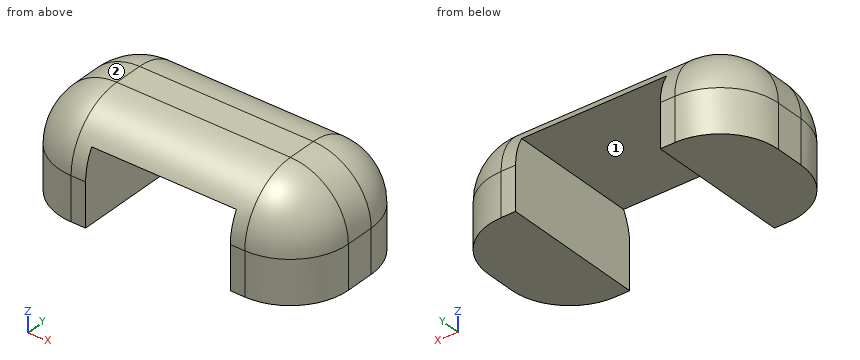
```python
from build123d import *

# Parameters (mm, degrees)
F0_W         = 5
F0_H         = 10
F1_DEPTH     = 5
F2_W         = 20
F2_H         = 10
F3_DEPTH     = 2
F4_T1_DEPTH  = 2
F4_T3_DEPTH  = 12
F4_T5_DEPTH  = 13
F4_S9_W      = 4
F4_S9_H      = 4
F4_T10_DEPTH = 4
F4_S15_W     = 4
F4_S15_H     = 4
F4_T16_DEPTH = 4
F4_S21_W     = 4
F4_S21_H     = 4
F4_T22_DEPTH = 4
F4_S27_W     = 4
F4_S27_H     = 4
F4_T28_DEPTH = 4


# Not quite as in the source:
# - a fillet or chamfer that OpenCascade refuses, or shapes differently, is made with other operations: its cross-section is extruded or revolved along the edge and cut away or added


with BuildPart() as f1:
    # F0 (on Top) → F1 (new body)
    with BuildSketch(Plane.XY):
        with Locations((-7.5, 0)):
            Rectangle(F0_W, F0_H)
    extrude(amount=F1_DEPTH)



with BuildPart() as f1b:
    # F0 (on Top) → F1, piece 2 (new body)
    with BuildSketch(Plane.XY):
        with Locations((7.5, 0)):
            Rectangle(F0_W, F0_H)
    extrude(amount=F1_DEPTH)


with BuildPart() as f1_1:
    add(f1.part)

    add(f1b.part)  # F3 merges F1b
    # F2 (on face) → F3 (join)
    with BuildSketch(Plane.XY.offset(5)):
        Rectangle(F2_W, F2_H)
    extrude(amount=F3_DEPTH)

    # F4: fillet of radius 4 on 8 edges, made by hand

    # F4_s2 → F4_t1 (cut)
    with BuildSketch(Plane.XZ.offset(-1)):
        with BuildLine():
            ThreePointArc((-10, 3), (-8.8284271247, 5.8284271247), (-6, 7))
            Line((-6, 7), (-10, 7))
            Line((-10, 7), (-10, 3))
        make_face()
        with BuildLine():
            ThreePointArc((6, 7), (8.8284271247, 5.8284271247), (10, 3))
            Line((10, 3), (10, 7))
            Line((10, 7), (6, 7))
        make_face()
    extrude(amount=F4_T1_DEPTH, mode=Mode.SUBTRACT)

    # F4_s4 → F4_t3 (cut)
    with BuildSketch(Plane.YZ.offset(-6)):
        with BuildLine():
            ThreePointArc((-5, 3), (-3.8284271247, 5.8284271247), (-1, 7))
            Line((-1, 7), (-5, 7))
            Line((-5, 7), (-5, 3))
        make_face()
        with BuildLine():
            ThreePointArc((5, 3), (3.8284271247, 5.8284271247), (1, 7))
            Line((1, 7), (5, 7))
            Line((5, 7), (5, 3))
        make_face()
    extrude(amount=F4_T3_DEPTH, mode=Mode.SUBTRACT)

    # F4_s6 → F4_t5 (cut)
    with BuildSketch(Plane.XY.offset(-10)):
        with BuildLine():
            ThreePointArc((6, -5), (8.8284271247, -3.8284271247), (10, -1))
            Line((10, -1), (10, -5))
            Line((10, -5), (6, -5))
        make_face()
        with BuildLine():
            ThreePointArc((6, 5), (8.8284271247, 3.8284271247), (10, 1))
            Line((10, 1), (10, 5))
            Line((10, 5), (6, 5))
        make_face()
        with BuildLine():
            ThreePointArc((-6, 5), (-8.8284271247, 3.8284271247), (-10, 1))
            Line((-10, 1), (-10, 5))
            Line((-10, 5), (-6, 5))
        make_face()
        with BuildLine():
            ThreePointArc((-6, -5), (-8.8284271247, -3.8284271247), (-10, -1))
            Line((-10, -1), (-10, -5))
            Line((-10, -5), (-6, -5))
        make_face()
    extrude(amount=F4_T5_DEPTH, mode=Mode.SUBTRACT)


with BuildPart() as f4_tool8:
    # F4_s9 → F4_t10 (new body)
    with BuildSketch(Plane.XY.offset(3)):
        with Locations((-8, 3)):
            Rectangle(F4_S9_W, F4_S9_H)
    extrude(amount=F4_T10_DEPTH)

    # F4_s11 → F4_t12 (revolve, cut)
    with BuildSketch(Plane(origin=(-6, 1, 3), x_dir=(0.7071067812, -0.7071067812, 0), z_dir=(-0.7071067812, -0.7071067812, 0))):
        with BuildLine():
            ThreePointArc((0, -4), (4, 0), (0, 4))
            Line((0, 4), (0, -4))
        make_face()
    revolve(axis=Axis((-6, 1, 3), (0, 0, 1)), mode=Mode.SUBTRACT)


with BuildPart() as f1_2:
    add(f1_1.part)

    # F4_t7: cut F4_tool8
    add(f4_tool8.part, mode=Mode.SUBTRACT)


with BuildPart() as f4_tool14:
    # F4_s15 → F4_t16 (new body)
    with BuildSketch(Plane.XY.offset(3)):
        with Locations((-8, -3)):
            Rectangle(F4_S15_W, F4_S15_H)
    extrude(amount=F4_T16_DEPTH)

    # F4_s17 → F4_t18 (revolve, cut)
    with BuildSketch(Plane(origin=(-6, -1, 3), x_dir=(0.7071067812, 0.7071067812, 0), z_dir=(0.7071067812, -0.7071067812, 0))):
        with BuildLine():
            ThreePointArc((0, -4), (4, 0), (0, 4))
            Line((0, 4), (0, -4))
        make_face()
    revolve(axis=Axis((-6, -1, 3), (0, 0, 1)), mode=Mode.SUBTRACT)


with BuildPart() as f1_3:
    add(f1_2.part)

    # F4_t13: cut F4_tool14
    add(f4_tool14.part, mode=Mode.SUBTRACT)


with BuildPart() as f4_tool20:
    # F4_s21 → F4_t22 (new body)
    with BuildSketch(Plane.XY.offset(3)):
        with Locations((8, -3)):
            Rectangle(F4_S21_W, F4_S21_H)
    extrude(amount=F4_T22_DEPTH)

    # F4_s23 → F4_t24 (revolve, cut)
    with BuildSketch(Plane(origin=(6, -1, 3), x_dir=(-0.7071067812, 0.7071067812, 0), z_dir=(0.7071067812, 0.7071067812, 0))):
        with BuildLine():
            ThreePointArc((0, -4), (4, 0), (0, 4))
            Line((0, 4), (0, -4))
        make_face()
    revolve(axis=Axis((6, -1, 3), (0, 0, 1)), mode=Mode.SUBTRACT)


with BuildPart() as f1_4:
    add(f1_3.part)

    # F4_t19: cut F4_tool20
    add(f4_tool20.part, mode=Mode.SUBTRACT)


with BuildPart() as f4_tool26:
    # F4_s27 → F4_t28 (new body)
    with BuildSketch(Plane.XY.offset(3)):
        with Locations((8, 3)):
            Rectangle(F4_S27_W, F4_S27_H)
    extrude(amount=F4_T28_DEPTH)

    # F4_s29 → F4_t30 (revolve, cut)
    with BuildSketch(Plane(origin=(6, 1, 3), x_dir=(-0.7071067812, -0.7071067812, 0), z_dir=(-0.7071067812, 0.7071067812, 0))):
        with BuildLine():
            ThreePointArc((0, -4), (4, 0), (0, 4))
            Line((0, 4), (0, -4))
        make_face()
    revolve(axis=Axis((6, 1, 3), (0, 0, 1)), mode=Mode.SUBTRACT)


with BuildPart() as f1_5:
    add(f1_4.part)

    # F4_t25: cut F4_tool26
    add(f4_tool26.part, mode=Mode.SUBTRACT)


solid = f1_5.part
```
The model under review builds one solid part; all positions refer to its coordinate system, in mm. Face numbers are marked on the shaded views. A direction names the side the tool comes from. Round coordinates to 2 decimals unless told otherwise and drop trailing zeros. Loops run counter-clockwise (first coordinate to the right, second up) from the corner with the lowest first, then second, coordinate; pieces in that order, holes last.
1) Clearance check with flat-ended pins moving along their axes: P1, Ø2, axis at x = 0.5, y = 2.5, coming from the +Z side; P2, Ø2, axis at x = 5, z = 4.5, coming from the -Y side; P3, Ø4, axis at y = -2, z = 2.5, coming from the +X side. State where each tip first meets the part, or that it passes through.
Values follow:
P1: stops at z = 6.97
P2: stops at y = -4.97
P3: stops at x = 10
2) Consider section D-D on z = 4. State the section outline as (x, y) points, then the cut area to 3 significant figures.
Values follow:
outline: (-9.87, -1) arc R3.87 ccw to (-6, -4.87) - (-5, -4.87) - (-5, 4.87) - (-6, 4.87) arc R3.87 ccw to (-9.87, 1) - close; (5, -4.87) - (6, -4.87) arc R3.87 ccw to (9.87, -1) - (9.87, 1) arc R3.87 ccw to (6, 4.87) - (5, 4.87) - close
area: 82.1 mm2
3) Consider section A-A on z = 1.25. State the section outline as (x, y) points, then the cut area to 3 significant figures.
Values follow:
outline: (-10, -1) arc R4 ccw to (-6, -5) - (-5, -5) - (-5, 5) - (-6, 5) arc R4 ccw to (-10, 1) - close; (5, -5) - (6, -5) arc R4 ccw to (10, -1) - (10, 1) arc R4 ccw to (6, 5) - (5, 5) - close
area: 86.3 mm2
4) Consider section B-B on y = 0. State the section outline as (x, z) points, then the cut area to 3 significant figures.
Values follow:
outline: (-10, 0) - (-5, 0) - (-5, 5) - (5, 5) - (5, 0) - (10, 0) - (10, 3) arc R4 ccw to (6, 7) - (-6, 7) arc R4 ccw to (-10, 3) - close
area: 83.1 mm2
5) Consider section C-C on x = -5.75. State the section outline as (y, z) points, then the cut area to 3 significant figures.
Values follow:
outline: (-5, 0) - (5, 0) - (5, 3) arc R4 ccw to (1, 7) - (-1, 7) arc R4 ccw to (-5, 3) - close
area: 63.1 mm2
6) Tool access review of the marked faces 1 and 2: name each direction out of +Z, -Z, +X, -X, +Y, -Y from which nothing blocks a thin tool from reaching the whole face with its end or side.
Values follow:
face 1: -Z, +Y, -Y
face 2: +Z, -X, +Y, -Y
7) Wall thickness on line 1 along X through (y, z) = (-1, 1.5); line 2 along X through (y, z) = (-2, 4.75); line 3 along Z through (x, y) = (2.75, -0.25): over which ranges is each line inside the solid? List them lowest first.
Values follow:
line 1: x = -10 to -5, 5 to 10
line 2: x = -9.46 to -5, 5 to 9.46
line 3: z = 5 to 7
